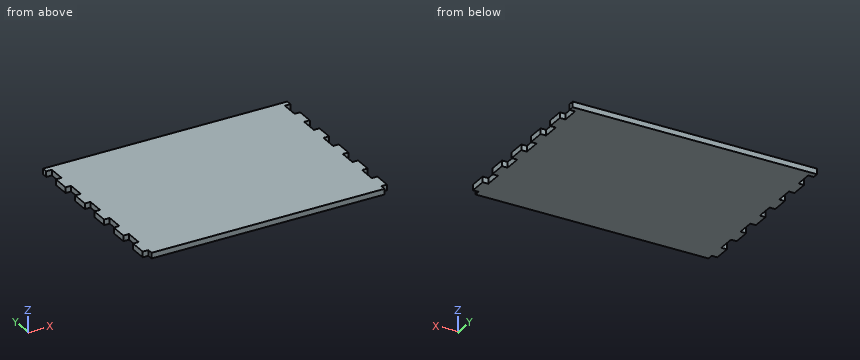
```python
from build123d import *

# Parameters (mm, degrees)
SKETCH1_W               = 276.86
SKETCH1_H               = 203.2
BOSS_EXTRUDE1_DEPTH     = 6.35
SKETCH2_W               = 6.35
SKETCH2_H               = 19.05
CUT_EXTRUDE1_DEPTH      = 172.830577605
LPATTERN1_COUNT         = 6
LPATTERN1_PITCH         = 38.1
MIRROR1_COPY_1_SKETCH_W = 6.35
MIRROR1_COPY_1_SKETCH_H = 19.05
MIRROR1_COPY_1_DEPTH    = 172.830577605
MIRROR1_COPY_2_SKETCH_W = 6.35
MIRROR1_COPY_2_SKETCH_H = 19.05
MIRROR1_COPY_2_DEPTH    = 172.830577605
MIRROR1_COPY_3_SKETCH_W = 6.35
MIRROR1_COPY_3_SKETCH_H = 19.05
MIRROR1_COPY_3_DEPTH    = 172.830577605
MIRROR1_COPY_4_SKETCH_W = 6.35
MIRROR1_COPY_4_SKETCH_H = 19.05
MIRROR1_COPY_4_DEPTH    = 172.830577605
MIRROR1_COPY_5_SKETCH_W = 6.35
MIRROR1_COPY_5_SKETCH_H = 19.05
MIRROR1_COPY_5_DEPTH    = 172.830577605


with BuildPart() as part:
    # Sketch1 → Boss-Extrude1 (new body)
    with BuildSketch(Plane.XY):
        Rectangle(SKETCH1_W, SKETCH1_H)
    extrude(amount=BOSS_EXTRUDE1_DEPTH)

    # Sketch2 → Cut-Extrude1 (cut, through all)
    with BuildSketch(Plane.XY.offset(6.35)):
        with Locations((-135.255, 85.725)):
            Rectangle(SKETCH2_W, SKETCH2_H)
    cut_extrude1 = extrude(amount=-CUT_EXTRUDE1_DEPTH, mode=Mode.SUBTRACT)

    # LPattern1: Cut-Extrude1 ×6
    with Locations(*[(0, -i * LPATTERN1_PITCH, 0) for i in range(1, LPATTERN1_COUNT)]):
        add(cut_extrude1, mode=Mode.SUBTRACT)

    # Mirror1: Cut-Extrude1 across plane
    add(cut_extrude1.mirror(Plane(origin=(0, 0, 0), x_dir=(0, 0, 1), z_dir=(1, 0, 0))), mode=Mode.SUBTRACT)

    # Mirror1 copy 1 sketch → Mirror1 copy 1 (cut, through all)
    with BuildSketch(Plane(origin=(0, -38.1, 6.35), x_dir=(-1, 0, 0), z_dir=(0, 0, 1))):
        with Locations((-135.255, -85.725)):
            Rectangle(MIRROR1_COPY_1_SKETCH_W, MIRROR1_COPY_1_SKETCH_H)
    extrude(amount=-MIRROR1_COPY_1_DEPTH, mode=Mode.SUBTRACT)

    # Mirror1 copy 2 sketch → Mirror1 copy 2 (cut, through all)
    with BuildSketch(Plane(origin=(0, -76.2, 6.35), x_dir=(-1, 0, 0), z_dir=(0, 0, 1))):
        with Locations((-135.255, -85.725)):
            Rectangle(MIRROR1_COPY_2_SKETCH_W, MIRROR1_COPY_2_SKETCH_H)
    extrude(amount=-MIRROR1_COPY_2_DEPTH, mode=Mode.SUBTRACT)

    # Mirror1 copy 3 sketch → Mirror1 copy 3 (cut, through all)
    with BuildSketch(Plane(origin=(0, -114.3, 6.35), x_dir=(-1, 0, 0), z_dir=(0, 0, 1))):
        with Locations((-135.255, -85.725)):
            Rectangle(MIRROR1_COPY_3_SKETCH_W, MIRROR1_COPY_3_SKETCH_H)
    extrude(amount=-MIRROR1_COPY_3_DEPTH, mode=Mode.SUBTRACT)

    # Mirror1 copy 4 sketch → Mirror1 copy 4 (cut, through all)
    with BuildSketch(Plane(origin=(0, -152.4, 6.35), x_dir=(-1, 0, 0), z_dir=(0, 0, 1))):
        with Locations((-135.255, -85.725)):
            Rectangle(MIRROR1_COPY_4_SKETCH_W, MIRROR1_COPY_4_SKETCH_H)
    extrude(amount=-MIRROR1_COPY_4_DEPTH, mode=Mode.SUBTRACT)

    # Mirror1 copy 5 sketch → Mirror1 copy 5 (cut, through all)
    with BuildSketch(Plane(origin=(0, -190.5, 6.35), x_dir=(-1, 0, 0), z_dir=(0, 0, 1))):
        with Locations((-135.255, -85.725)):
            Rectangle(MIRROR1_COPY_5_SKETCH_W, MIRROR1_COPY_5_SKETCH_H)
    extrude(amount=-MIRROR1_COPY_5_DEPTH, mode=Mode.SUBTRACT)


solid = part.part
```
The listing builds one solid part. Answer for the finished solid, in the listing's coordinates (mm). Give positions to 0.01 mm unless a question says otherwise; leave off trailing zeros. Order: outer loops, then holes, each group sorted by start corner. A loop starts at its lowest first (then second) coordinate and runs counter-clockwise, first axis right, second up. Notation, with made-up numbers: (-5, 46) -> (47, 46) arc R15 cw to (47, 73) -> close; hole circle Ø6 at (-9.5, 35). An arc over 180 degrees is marked (long way). Answer as a JSON object with one key per item and string values. Group by question number.
Item 1: Consider L1, parallel to X at y = -35.5, z = 0.75. Determine where the line is inside the solid, lowest interval first. Write a range as from..to.
Item 2: The part is cut by section A-A on y = 44. Write down the section's boundary in (x, z), and give its area (3 significant figures).
Item 3: Flat-ended cylindrical pins translate along their axes: pin 1 (2 mm diameter, centred on y = -30, z = 3.5, fed in from +X); pin 2 (3 mm diameter, centred on x = -136.5, z = 1.5, fed in from -Y). Find the tip coordinate at first contact, or state that the pin passes through.
Result set:
{
 "1": {"L1": "-132.08..132.08"},
 "2": {"outline": "(-132.08, 0) -> (132.08, 0) -> (132.08, 6.35) -> (-132.08, 6.35) -> close", "area": "1,680 mm²"},
 "3": {"pin 1": "x = 132.08", "pin 2": "y = -95.25"}
}
